Input: part model. Units: mm. Frame: model coordinates. Give positions to 0.01 mm unless a question says otherwise; leave off trailing zeros. Loops run counter-clockwise (first coordinate to the right, second up) from the corner with the lowest first, then second, coordinate; pieces in that order, holes last. Notation, with made-up numbers: M 57.5,77.25 L 64.5,77.25 A21 ccw 64.5,95.25 Z; hole C -16,-18.75 d2. An arc over 180 degrees is marked long. Answer as a JSON object with one key per item and string values. Group by question number.
1) Ray query, L1, parallel to X at y = 262.5, z = 21; L2, parallel to X at y = 76, z = 16. Return the intervals inside material, ascending.
2) Section query B-B on z = 8.5. Count the separate pieces of the cut face and the enclosed holes in it, plus the area to 3 significant figures.
3) Section query A-A on y = 255. Return loops of the section in (x, z), plus the area to 4 significant figures.
4) Draft query along Y for faces 1 (the flat face through (-1, 700, 12)), 2 (the cylindrical face through (-3.06, 193.3, 12.32)), 3 (the flat face through (100, -10, 12)), 4 (the cylindrical face through (-5.094, 572.059, 12.325)). Return one class per face: +Y half, -Y half, draft (parallel to the pull), parting line (faces both ways), or undercut.
from build123d import *

# Parameters (mm, degrees)
F0_W     = 200
F0_H     = 1400
F0_R     = 2.5
F0_R_2   = 23.5
F1_DEPTH = 25


with BuildPart() as f1:
    # F0 (on Top) → F1 (new body)
    with BuildSketch(Plane.XY):
        Rectangle(F0_W, F0_H)
        with Locations((-21.213203, -616.213203)):
            Circle(F0_R, mode=Mode.SUBTRACT)
        with Locations((-21.213203, -573.786797)):
            Circle(F0_R, mode=Mode.SUBTRACT)
        with Locations((-21.213203, -531.213203)):
            Circle(F0_R, mode=Mode.SUBTRACT)
        with Locations((-21.213203, -488.786797)):
            Circle(F0_R, mode=Mode.SUBTRACT)
        with Locations((-21.213203, -446.213203)):
            Circle(F0_R, mode=Mode.SUBTRACT)
        with Locations((-21.213203, -403.786797)):
            Circle(F0_R, mode=Mode.SUBTRACT)
        with Locations((-21.213203, -361.213203)):
            Circle(F0_R, mode=Mode.SUBTRACT)
        with Locations((-21.213203, -318.786797)):
            Circle(F0_R, mode=Mode.SUBTRACT)
        with Locations((-21.213203, -276.213203)):
            Circle(F0_R, mode=Mode.SUBTRACT)
        with Locations((-21.213203, -233.786797)):
            Circle(F0_R, mode=Mode.SUBTRACT)
        with Locations((-21.213203, -191.213203)):
            Circle(F0_R, mode=Mode.SUBTRACT)
        with Locations((-21.213203, -148.786797)):
            Circle(F0_R, mode=Mode.SUBTRACT)
        with Locations((-21.213203, -106.213203)):
            Circle(F0_R, mode=Mode.SUBTRACT)
        with Locations((-21.213203, -63.786797)):
            Circle(F0_R, mode=Mode.SUBTRACT)
        with Locations((-21.213203, -21.213203)):
            Circle(F0_R, mode=Mode.SUBTRACT)
        with Locations((21.213203, -616.213203)):
            Circle(F0_R, mode=Mode.SUBTRACT)
        with Locations((0, -595)):
            Circle(F0_R_2, mode=Mode.SUBTRACT)
        with Locations((21.213203, -573.786797)):
            Circle(F0_R, mode=Mode.SUBTRACT)
        with Locations((21.213203, -531.213203)):
            Circle(F0_R, mode=Mode.SUBTRACT)
        with Locations((0, -510)):
            Circle(F0_R_2, mode=Mode.SUBTRACT)
        with Locations((21.213203, -488.786797)):
            Circle(F0_R, mode=Mode.SUBTRACT)
        with Locations((21.213203, -446.213203)):
            Circle(F0_R, mode=Mode.SUBTRACT)
        with Locations((0, -425)):
            Circle(F0_R_2, mode=Mode.SUBTRACT)
        with Locations((21.213203, -403.786797)):
            Circle(F0_R, mode=Mode.SUBTRACT)
        with Locations((21.213203, -361.213203)):
            Circle(F0_R, mode=Mode.SUBTRACT)
        with Locations((0, -340)):
            Circle(F0_R_2, mode=Mode.SUBTRACT)
        with Locations((21.213203, -318.786797)):
            Circle(F0_R, mode=Mode.SUBTRACT)
        with Locations((21.213203, -276.213203)):
            Circle(F0_R, mode=Mode.SUBTRACT)
        with Locations((0, -255)):
            Circle(F0_R_2, mode=Mode.SUBTRACT)
        with Locations((21.213203, -233.786797)):
            Circle(F0_R, mode=Mode.SUBTRACT)
        with Locations((21.213203, -191.213203)):
            Circle(F0_R, mode=Mode.SUBTRACT)
        with Locations((0, -170)):
            Circle(F0_R_2, mode=Mode.SUBTRACT)
        with Locations((21.213203, -148.786797)):
            Circle(F0_R, mode=Mode.SUBTRACT)
        with Locations((21.213203, -106.213203)):
            Circle(F0_R, mode=Mode.SUBTRACT)
        with Locations((0, -85)):
            Circle(F0_R_2, mode=Mode.SUBTRACT)
        with Locations((21.213203, -63.786797)):
            Circle(F0_R, mode=Mode.SUBTRACT)
        with Locations((21.213203, -21.213203)):
            Circle(F0_R, mode=Mode.SUBTRACT)
        with Locations((-21.213203, 21.213203)):
            Circle(F0_R, mode=Mode.SUBTRACT)
        with Locations((-21.213203, 63.786797)):
            Circle(F0_R, mode=Mode.SUBTRACT)
        with Locations((-21.213203, 106.213203)):
            Circle(F0_R, mode=Mode.SUBTRACT)
        with Locations((-21.213203, 148.786797)):
            Circle(F0_R, mode=Mode.SUBTRACT)
        with Locations((-21.213203, 191.213203)):
            Circle(F0_R, mode=Mode.SUBTRACT)
        with Locations((-21.213203, 233.786797)):
            Circle(F0_R, mode=Mode.SUBTRACT)
        with Locations((-21.213203, 276.213203)):
            Circle(F0_R, mode=Mode.SUBTRACT)
        with Locations((-21.213203, 318.786797)):
            Circle(F0_R, mode=Mode.SUBTRACT)
        with Locations((-21.213203, 361.213203)):
            Circle(F0_R, mode=Mode.SUBTRACT)
        with Locations((-21.213203, 403.786797)):
            Circle(F0_R, mode=Mode.SUBTRACT)
        with Locations((-21.213203, 446.213203)):
            Circle(F0_R, mode=Mode.SUBTRACT)
        with Locations((-21.213203, 488.786797)):
            Circle(F0_R, mode=Mode.SUBTRACT)
        with Locations((-21.213203, 531.213203)):
            Circle(F0_R, mode=Mode.SUBTRACT)
        with Locations((-21.213203, 573.786797)):
            Circle(F0_R, mode=Mode.SUBTRACT)
        with Locations((-21.213203, 616.213203)):
            Circle(F0_R, mode=Mode.SUBTRACT)
        Circle(F0_R_2, mode=Mode.SUBTRACT)
        with Locations((0, 85)):
            Circle(F0_R_2, mode=Mode.SUBTRACT)
        with Locations((21.213203, 21.213203)):
            Circle(F0_R, mode=Mode.SUBTRACT)
        with Locations((21.213203, 63.786797)):
            Circle(F0_R, mode=Mode.SUBTRACT)
        with Locations((0, 170)):
            Circle(F0_R_2, mode=Mode.SUBTRACT)
        with Locations((21.213203, 106.213203)):
            Circle(F0_R, mode=Mode.SUBTRACT)
        with Locations((21.213203, 148.786797)):
            Circle(F0_R, mode=Mode.SUBTRACT)
        with Locations((0, 255)):
            Circle(F0_R_2, mode=Mode.SUBTRACT)
        with Locations((21.213203, 191.213203)):
            Circle(F0_R, mode=Mode.SUBTRACT)
        with Locations((21.213203, 233.786797)):
            Circle(F0_R, mode=Mode.SUBTRACT)
        with Locations((0, 340)):
            Circle(F0_R_2, mode=Mode.SUBTRACT)
        with Locations((21.213203, 276.213203)):
            Circle(F0_R, mode=Mode.SUBTRACT)
        with Locations((21.213203, 318.786797)):
            Circle(F0_R, mode=Mode.SUBTRACT)
        with Locations((0, 425)):
            Circle(F0_R_2, mode=Mode.SUBTRACT)
        with Locations((21.213203, 361.213203)):
            Circle(F0_R, mode=Mode.SUBTRACT)
        with Locations((21.213203, 403.786797)):
            Circle(F0_R, mode=Mode.SUBTRACT)
        with Locations((0, 510)):
            Circle(F0_R_2, mode=Mode.SUBTRACT)
        with Locations((21.213203, 446.213203)):
            Circle(F0_R, mode=Mode.SUBTRACT)
        with Locations((21.213203, 488.786797)):
            Circle(F0_R, mode=Mode.SUBTRACT)
        with Locations((0, 595)):
            Circle(F0_R_2, mode=Mode.SUBTRACT)
        with Locations((21.213203, 531.213203)):
            Circle(F0_R, mode=Mode.SUBTRACT)
        with Locations((21.213203, 573.786797)):
            Circle(F0_R, mode=Mode.SUBTRACT)
        with Locations((21.213203, 616.213203)):
            Circle(F0_R, mode=Mode.SUBTRACT)
    extrude(amount=F1_DEPTH)


solid = f1.part
Output:
{
 "1": {"L1": "x = -100 to -22.27, 22.27 to 100", "L2": "x = -100 to -21.71, 21.71 to 100"},
 "2": {"separate pieces": "1", "enclosed holes": "75", "area": "253,000 mm^2"},
 "3": {"outline": "M -100,0 L -23.5,0 L -23.5,25 L -100,25 Z; M 23.5,0 L 100,0 L 100,25 L 23.5,25 Z", "area": "3,825 mm^2"},
 "4": {"face 1": "+Y half", "face 2": "undercut", "face 3": "draft", "face 4": "undercut"}
}
